Geometry check sheet. Reference: drawing and pictorial views, mm from the part's lowest x, y, z. A direction names the side the tool comes from. Give positions to 0.01 mm unless a question says otherwise; leave off trailing zeros. Loops run counter-clockwise (first coordinate to the right, second up) from the corner with the lowest first, then second, coordinate; pieces in that order, holes last. Notation, with made-up numbers: (-32, 6) - (16, 6) arc R9 ccw to (16, 18) - close; hole circle Ø5 at (46, 11). An arc over 180 degrees is marked (long way). Answer in a Markdown table with one row per item. Add a question column.
(1) Sectioned sample at D-D on z = 19.25. Enter the section's corners in (x, y).
(2) Sectioned sample at B-B on x = 14. Enter the section's corners in (y, z).
(3) Draft check along X on the marked faces 4, 5 and 6. Enter one of: released by +X, released by -X, zero draft, split by the parting line, or undercut.
(4) Set-up check for the marked faces 1, 2 and 3: record each of +Z, -Z, +X, -X, +Y, -Y from which the full face is reachable in a straight line by a thin tool's end or side.
(5) Thickness scan on L1, parallel to Y at x = 20.25, z = 14; L2, parallel to Z at x = 13.75, y = 6.75; L3, parallel to Y at x = 19, z = 11.5. Record the ranges inside material, lowest first.
(6) Sectioned sample at A-A on y = 4.5. Enter the section's corners in (x, z), then the cut area to 3 significant figures.
(7) Go/stop test with flat-tipped pins: P1, Ø2, axis at x = 21, y = 6, coming from the -Z side; P2, Ø6, axis at x = 17.5, z = 19.5, coming from the +Y side; P3, Ø2, axis at y = 3.5, z = 5.5, coming from the +X side. Record where each tip stops, or that it passes through.
(8) Sectioned sample at C-C on z = 14. Enter the section's corners in (x, y), then the cut area to 3 significant figures.
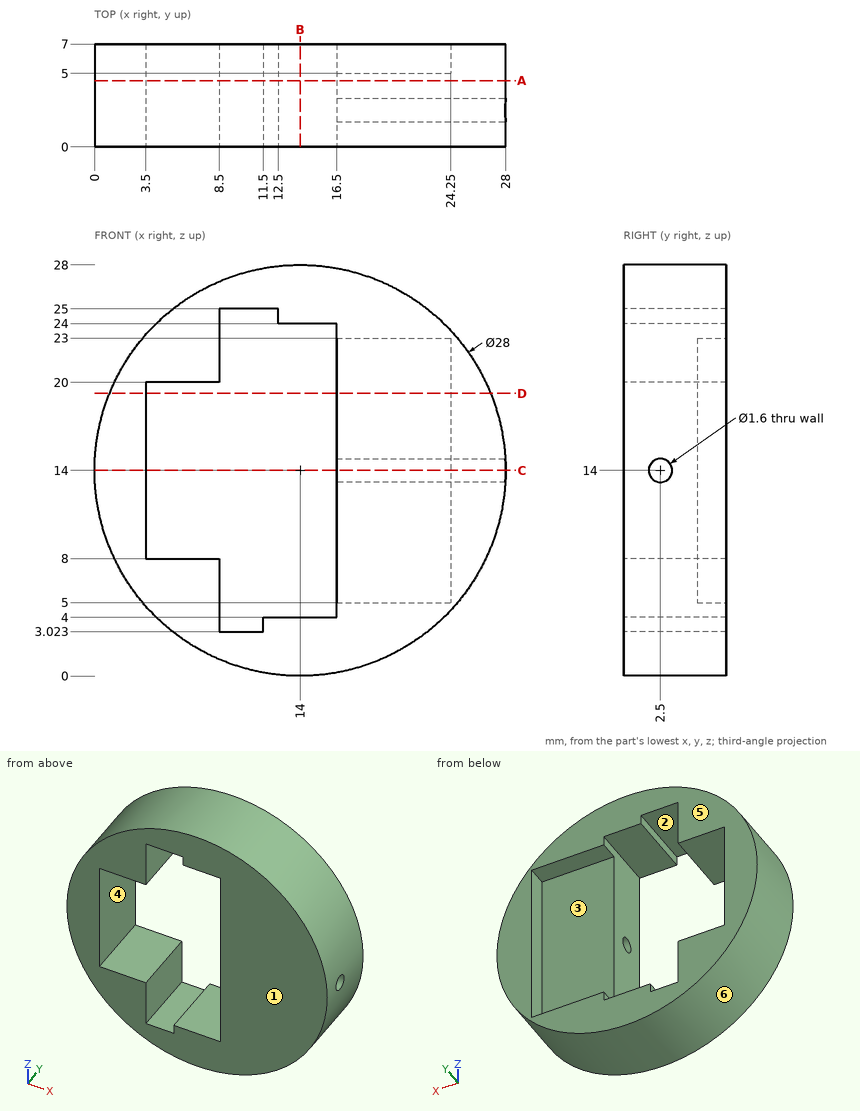
Reply:
| question | item | result |
|---|---|---|
| 1 | outline | (1.02, 0) - (3.5, 0) - (3.5, 7) - (1.02, 7) - close; (16.5, 0) - (26.98, 0) - (26.98, 7) - (24.25, 7) - (24.25, 5) - (16.5, 5) - close |
| 2 | outline | (0, 0) - (7, 0) - (7, 4) - (0, 4) - close; (0, 24) - (7, 24) - (7, 28) - (0, 28) - close |
| 3 | face 4 | undercut |
| 3 | face 5 | zero draft |
| 3 | face 6 | split by the parting line |
| 4 | face 1 | +Z, -Z, +X, -X, -Y |
| 4 | face 2 | +Y, -Y |
| 4 | face 3 | +Y |
| 5 | L1 | 0 to 1.7, 3.3 to 5 |
| 5 | L2 | 0 to 4, 24 to 28 |
| 5 | L3 | 0 to 5 |
| 6 | outline | circle Ø28 at (14, 14); hole (3.5, 8) - (8.5, 8) - (8.5, 3.02) - (11.5, 3.02) - (11.5, 4) - (16.5, 4) - (16.5, 24) - (12.5, 24) - (12.5, 25) - (8.5, 25) - (8.5, 20) - (3.5, 20) - close |
| 6 | area | 389 mm^2 |
| 7 | P1 | z = 1.35 |
| 7 | P2 | y = 5 |
| 7 | P3 | x = 25.82 |
| 8 | outline | (0, 0) - (3.5, 0) - (3.5, 7) - (0, 7) - close; (16.5, 0) - (28, 0) - (28, 1.7) - (16.5, 1.7) - close; (16.5, 3.3) - (28, 3.3) - (28, 7) - (24.25, 7) - (24.25, 5) - (16.5, 5) - close |
| 8 | area | 71.1 mm^2 |
